from build123d import *
from OCP.BRepFilletAPI import BRepFilletAPI_MakeChamfer

# Parameters (mm, degrees)
SKETCH1_W           = 22.8
SKETCH1_H           = 30
BOSS_EXTRUDE1_DEPTH = 11.6
SKETCH3_W           = 4.25
SKETCH3_H           = 2.1
BOSS_EXTRUDE2_DEPTH = 11.6
SKETCH4_R           = 1
CUT_EXTRUDE1_DEPTH  = 11.6
SKETCH2_R           = 1
CUT_EXTRUDE2_DEPTH  = 5
CHAMFER1_SIZE       = 5
CHAMFER1_SIZE2      = 3.63271264


with BuildPart() as part:
    # Sketch1 → Boss-Extrude1 (new body)
    with BuildSketch(Plane.XY):
        Rectangle(SKETCH1_W, SKETCH1_H)
    extrude(amount=BOSS_EXTRUDE1_DEPTH)

    # Sketch3 → Boss-Extrude2 (add)
    with BuildSketch(Plane.XY.offset(11.6)):
        with Locations((-13.525, 6.55)):
            Rectangle(SKETCH3_W, SKETCH3_H)
        with Locations((13.525, 6.55)):
            Rectangle(SKETCH3_W, SKETCH3_H)
    extrude(amount=-BOSS_EXTRUDE2_DEPTH)

    # Sketch4 → Cut-Extrude1 (cut)
    with BuildSketch(Plane(origin=(0, 7.6, 0), x_dir=(1, 0, 0), z_dir=(0, 1, 0))):
        with Locations(Location((-14, -5.8, 0), (0, 0, 180))):
            Circle(SKETCH4_R)
        with Locations(Location((14, -5.8, 0), (0, 0, 90))):
            Circle(SKETCH4_R)
    extrude(amount=-CUT_EXTRUDE1_DEPTH, mode=Mode.SUBTRACT)

    # Sketch2 → Cut-Extrude2 (cut)
    with BuildSketch(Plane(origin=(0, 15, 0), x_dir=(1, 0, 0), z_dir=(0, 1, 0))):
        with Locations(Location((-5.4, -5.8, 0), (0, 0, 270))):
            Circle(SKETCH2_R)
    extrude(amount=-CUT_EXTRUDE2_DEPTH, mode=Mode.SUBTRACT)

    # Chamfer1: one chamfer whose edges measure the first distance from different faces: ONE call of the kernel's chamfer builder (chamfer() names one face for all edges)
    chamfer1_edges_1 = [part.edges().sort_by_distance(p)[0] for p in [
        (-11.4, 15, 5.8),
    ]]
    chamfer1_side_1 = [part.faces().sort_by_distance(p)[0] for p in [
        (-11.4, 11.3, 5.8),
    ]]
    chamfer1_edges_2 = [part.edges().sort_by_distance(p)[0] for p in [
        (11.4, 15, 5.8),
    ]]
    chamfer1_side_2 = [part.faces().sort_by_distance(p)[0] for p in [
        (11.4, 11.3, 5.8),
    ]]
    chamfer1 = BRepFilletAPI_MakeChamfer(part.part.solid().wrapped)
    for e in chamfer1_edges_1:
        chamfer1.Add(CHAMFER1_SIZE, CHAMFER1_SIZE2, e.wrapped, chamfer1_side_1[0].wrapped)  # the first distance lies on this face
    for e in chamfer1_edges_2:
        chamfer1.Add(CHAMFER1_SIZE, CHAMFER1_SIZE2, e.wrapped, chamfer1_side_2[0].wrapped)  # the first distance lies on this face
    add(Compound.cast(chamfer1.Shape()), mode=Mode.REPLACE)


solid = part.part
Geometry: final body of the model. Coordinates: model frame, mm. A direction names the side the tool comes from. Coordinates: 2 decimals unless noted, no trailing zeros. Order: outer loops, then holes, each group sorted by start corner. A loop starts at its lowest first (then second) coordinate and runs counter-clockwise, first axis right, second up.
(1) Access query for faces 4 (the face through (-11.4, 9, 6)), 5 (the face through (12.6, 7.6, 5.9)), 6 (the face through (-12.6, 5.5, 5.9)), 7 (the face through (12.6, 5.5, 5.9)). Directions: +Z, -Z, +X, -X, +Y, -Y. A direction counts if a zero-diameter tool reaches every point of the face in a straight line with its end or side. Return the directions, or none.
(2) Material intervals for probe 1 along Z at (x, y) = (-14, 6.75); probe 2 along X at (y, z) = (-12.25, 5.5); probe 3 along Y at (x, z) = (-12, 7.75), sorted ascending.
(3) Draft query along Z for faces 1 (the face through (-11.4, -5, 6)), 2 (the face through (-5, 10, 6)), 3 (the face through (0, 0, 11.6)). Return one class per face: pulls with the +Z half, pulls with the -Z half, needs draft (parallel to the pull), parting line crosses it, or undercut.
(4) Section query A-A (x = 14). Return the cut outline in (y, z).
(5) Section query D-D (x = -5.4). Return the cut outline in (y, z), plus the area to 3 significant figures.
(6) Section query B-B (z = 5.8). Return the cut outline in (x, y), plus the area to 3 significant figures.
(7) First-contact query: pin 1 (2 mm diameter, centred on x = 13.5, z = 7, fed in from +Y); pin 2 (3.5 mm diameter, centred on x = -13.5, z = 4, fed in from -Y); pin 3 (6 mm diameter, centred on y = -4, z = 4.5, fed in from +X); pin 4 (3 mm diameter, centred on x = 7, y = -8.5, fed in from -Z). Flat tips, straight axial feed; report the tip coordinate or a pass-through.
(8) Section query C-C (z = 4). Return the cut outline in (x, y).
Solution:
1. face 4: +Z, -Z, -X, +Y
1. face 5: +Z, -Z, +X, +Y
1. face 6: +Z, -Z, -X, -Y
1. face 7: +Z, -Z, +X, -Y
2. probe 1: z = 0 to 4.8, 6.8 to 11.6
2. probe 2: x = -11.4 to 11.4
2. probe 3: y = 5.5 to 7.6
3. face 1: needs draft
3. face 2: undercut
3. face 3: pulls with the +Z half
4. outline: (5.5, 0) - (7.6, 0) - (7.6, 4.8) - (5.5, 4.8) - close; (5.5, 6.8) - (7.6, 6.8) - (7.6, 11.6) - (5.5, 11.6) - close
5. outline: (-15, 0) - (15, 0) - (15, 4.8) - (10, 4.8) - (10, 6.8) - (15, 6.8) - (15, 11.6) - (-15, 11.6) - close
5. area: 338 mm2
6. outline: (-15.65, 5.5) - (-15, 5.5) - (-15, 7.6) - (-15.65, 7.6) - close; (-13, 5.5) - (-11.4, 5.5) - (-11.4, -15) - (11.4, -15) - (11.4, 5.5) - (13, 5.5) - (13, 7.6) - (11.4, 7.6) - (11.4, 10) - (7.77, 15) - (-4.4, 15) - (-4.4, 10) - (-6.4, 10) - (-6.4, 15) - (-7.77, 15) - (-11.4, 10) - (-11.4, 7.6) - (-13, 7.6) - close; (15, 5.5) - (15.65, 5.5) - (15.65, 7.6) - (15, 7.6) - close
6. area: 665 mm2
7. pin 1: stops at y = 7.6
7. pin 2: stops at y = 5.5
7. pin 3: stops at x = 11.4
7. pin 4: stops at z = 0
8. outline: (-15.65, 5.5) - (-11.4, 5.5) - (-11.4, -15) - (11.4, -15) - (11.4, 5.5) - (15.65, 5.5) - (15.65, 7.6) - (11.4, 7.6) - (11.4, 10) - (7.77, 15) - (-7.77, 15) - (-11.4, 10) - (-11.4, 7.6) - (-15.65, 7.6) - close
